Part model, mm, in its own coordinate system. Face numbers are marked on the shaded views. A direction names the side the tool comes from. Round coordinates to 2 decimals unless told otherwise and drop trailing zeros. Loops run counter-clockwise (first coordinate to the right, second up) from the corner with the lowest first, then second, coordinate; pieces in that order, holes last. Notation, with made-up numbers: M 12.5,-1 L 60.5,-1 A18 ccw 60.5,32 Z; hole C -2,28.25 d11. An arc over 180 degrees is marked long. Put each result on its own line as item: value. Start each with the question number.
1) Which spindle directions (+Z, -Z, +X, -X, +Y, -Y) get a long thin tool onto all of the face, cutting with end or side? Do the marked faces 4 and 5. Say none if no direction does.
2) Slice it at D-D on y = 83.5. Give the cut face in (x, z), then the cut area to 3 significant figures.
3) Pull direction Y, two halves, no side cores. Call the marked faces 1, 2 and 3: +Y half, -Y half, draft (parallel to the pull), parting line (faces both ways), or undercut.
4) Probe line 1 along Y through (x, z) = (-89.5, 19.5); line 2 along X through (y, z) = (78.5, 4); line 3 along Z through (x, y) = (-70, 52). List the from-to ranges inside material, lowest first.
5) Drop flat-ended pins along their axis: pin 1 Ø8 at (y, z) = (-19, 20.5) entering from +X; pin 2 Ø3 at (y, z) = (34, 16) entering from -X; pin 3 Ø10 at (x, y) = (-54, 29) entering from +Z; pin 4 Ø11 at (x, y) = (83.15, 34.44) entering from +Z. Give the stop position or say it passes through.
6) Slice it at C-C on z = 10. State how many separate pieces and enclosed holes the cut face has, then the cut area to 3 significant figures.
```python
from build123d import *

# Parameters (mm, degrees)
F3_DEPTH        = 20.001
F3_COPIES_COUNT = 8
F6_R            = 8


# Not quite as in the source:
# - a pattern or mirror of a feature is missing from the dataset's text; its kind, count and spacing are read off the source's solid


with BuildPart() as f1:
    # F0 (on Front) → F1 (revolve)
    with BuildSketch(Plane.XZ):
        Polygon((54, 52), (54, 0), (79, 0), (79, 2), (110, 2), (110, 20), (65.5, 20), (57.15, 40), (57.15, 52), align=None)
    revolve(axis=Axis((0, 0, 26), (0, 0, -1)))

    # F2 (on face) → F3 (cut, through all)
    with BuildSketch(Plane.XY.offset(20)):
        with BuildLine():
            ThreePointArc((74.8342421334, 30.9973580216), (84.9049708242, 25.6144413892), (92.149157926, 34.4415089129))
            ThreePointArc((92.149157926, 34.4415089129), (81.3933450279, 43.2685764365), (74.8342421334, 30.9973580216))
        make_face()
    f3 = extrude(amount=-F3_DEPTH, mode=Mode.SUBTRACT)

    # F3_copies: F3 ×8 about axis
    f3_copies_axis = Axis((0, 0, 0), (0, 0, 1))
    for i in range(1, F3_COPIES_COUNT):
        add(f3.rotate(f3_copies_axis, i * 360 / F3_COPIES_COUNT), mode=Mode.SUBTRACT)

    # F4 (on Front) → F5 (revolve, cut)
    with BuildSketch(Plane.XZ):
        Polygon((57.15, 52), (55, 52), (55, 51.999), (57.15, 50.3492469758), align=None)
    revolve(axis=Axis((0, 0, 26), (0, 0, -1)), mode=Mode.SUBTRACT)

    # F6
    f6_edges = [f1.edges().sort_by_distance(p)[0] for p in [
        (-65.5, 0, 20),
    ]]
    fillet(f6_edges, radius=F6_R)


solid = f1.part
```
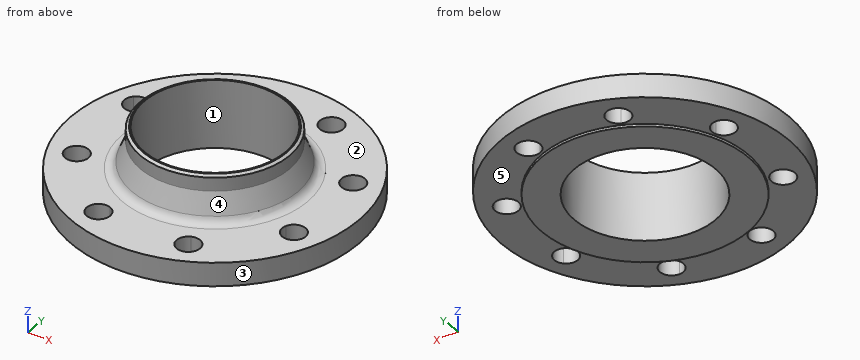
Recorded:
1. face 4: +Z
1. face 5: -Z
2. outline: M -71.61,2 L -43.43,2 L -43.43,20 L -71.61,20 Z; M -25.45,2 L 25.45,2 L 25.45,20 L -25.45,20 Z; M 43.43,2 L 71.61,2 L 71.61,20 L 43.43,20 Z
2. area: 1,930 mm2
3. face 1: undercut
3. face 2: draft
3. face 3: parting line
4. line 1: y = -63.95 to -40.82, -28.06 to 28.06, 40.82 to 63.95
4. line 2: x = -77.06 to -42.15, -26.74 to 26.74, 42.15 to 77.06
4. line 3: z = 2 to 20
5. pin 1: stops at x = 108.97
5. pin 2: stops at x = -105.09
5. pin 3: stops at z = 51.01
5. pin 4: passes through
6. separate pieces: 1
6. enclosed holes: 9
6. area: 26,800 mm2
